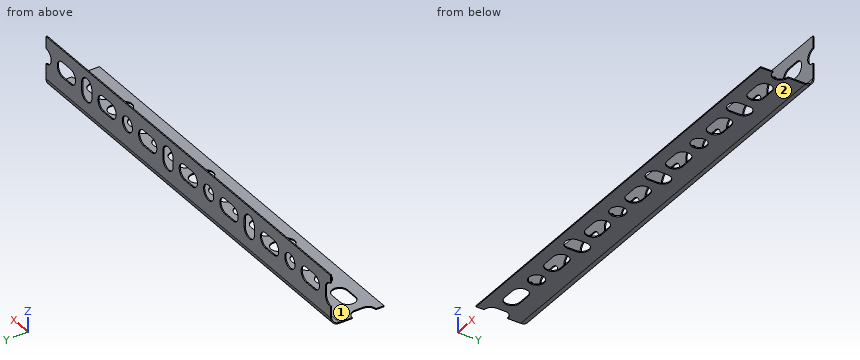
```python
from build123d import *

# Parameters (mm, degrees)
SKETCH1_W                    = 280
SKETCH1_H                    = 0.7366
BASE_FLANGE1_DEPTH           = 35
EDGE_FLANGE1_STRIP_W         = 12.9464
EDGE_FLANGE1_STRIP_H         = 0.7366
EDGE_FLANGE1_STRIP_CUT_DEPTH = 280
EDGE_FLANGE1_DEPTH           = 280
SKETCH11_R                   = 5
CUT_EXTRUDE1_DEPTH           = 149.199723952
LPATTERN1_COUNT              = 14
LPATTERN1_PITCH              = 80
SKETCH12_R                   = 5
CUT_EXTRUDE2_DEPTH           = 35
LPATTERN2_COUNT              = 15
LPATTERN2_PITCH              = 80


# Sheet-metal steps are written as plain solids
with BuildPart() as part:
    # Sketch1 → Base-Flange1 (new body)
    with BuildSketch(Plane(origin=(0, 0, 0), x_dir=(1, 0, 0), z_dir=(0, 1, 0))):
        with Locations((0, -0.3683)):
            Rectangle(SKETCH1_W, SKETCH1_H)
    extrude(amount=BASE_FLANGE1_DEPTH)

    # Edge-Flange1 strip (across the edge) → Edge-Flange1 strip cut (cut)
    with BuildSketch(Plane(origin=(140, 35, 0.7366), x_dir=(0, -1, 0), z_dir=(-1, 0, 0))):
        with Locations((-0.7366, -0.3683)):
            Rectangle(EDGE_FLANGE1_STRIP_W, EDGE_FLANGE1_STRIP_H)
    extrude(amount=EDGE_FLANGE1_STRIP_CUT_DEPTH, mode=Mode.SUBTRACT)

    # Edge-Flange1 section (across the edge) → Edge-Flange1 (add)
    with BuildSketch(Plane(origin=(140, 35, 0.7366), x_dir=(0, -1, 0), z_dir=(-1, 0, 0))):
        with BuildLine():
            Line((0, 5), (0, 33))
            Line((0, 33), (0.7366, 33))
            Line((0.7366, 33), (0.7366, 5))
            ThreePointArc((0.7366, 5), (2.201066094, 1.464466094), (5.7366, 0))
            Line((5.7366, 0), (5.7366, -0.7366))
            ThreePointArc((5.7366, -0.7366), (1.680211239, 0.943611239), (0, 5))
        make_face()
    extrude(amount=EDGE_FLANGE1_DEPTH)

    # Sketch11 → Cut-Extrude1 (cut, through all)
    with BuildSketch(Plane(origin=(0, 35, 0), x_dir=(1, 0, 0), z_dir=(0, 1, 0))):
        with Locations((140, -20.7366)):
            Circle(SKETCH11_R)
        with BuildLine():
            Line((124, -25.7366), (116, -25.7366))
            ThreePointArc((116, -25.7366), (111, -20.7366), (116, -15.7366))
            Line((116, -15.7366), (124, -15.7366))
            ThreePointArc((124, -15.7366), (129, -20.7366), (124, -25.7366))
        make_face()
        with BuildLine():
            Line((84, -25.7366), (76, -25.7366))
            ThreePointArc((76, -25.7366), (71, -20.7366), (76, -15.7366))
            Line((76, -15.7366), (84, -15.7366))
            ThreePointArc((84, -15.7366), (89, -20.7366), (84, -25.7366))
        make_face()
        with BuildLine():
            Line((95, -23.4866), (95, -17.9866))
            ThreePointArc((95, -17.9866), (100, -12.9866), (105, -17.9866))
            Line((105, -17.9866), (105, -23.4866))
            ThreePointArc((105, -23.4866), (100, -28.4866), (95, -23.4866))
        make_face()
    cut_extrude1 = extrude(amount=-CUT_EXTRUDE1_DEPTH, mode=Mode.SUBTRACT)

    # LPattern1: Cut-Extrude1 ×14
    with Locations(*[(-i * LPATTERN1_PITCH, 0, 0) for i in range(1, LPATTERN1_COUNT)]):
        add(cut_extrude1, mode=Mode.SUBTRACT)

    # Sketch12 → Cut-Extrude2 (cut)
    with BuildSketch(Plane.XY.offset(0.7366)):
        with Locations((140, 13)):
            Circle(SKETCH12_R)
        with BuildLine():
            Line((124, 8), (116, 8))
            ThreePointArc((116, 8), (111, 13), (116, 18))
            Line((116, 18), (124, 18))
            ThreePointArc((124, 18), (129, 13), (124, 8))
        make_face()
        with BuildLine():
            Line((95, 10.25), (95, 15.75))
            ThreePointArc((95, 15.75), (100, 20.75), (105, 15.75))
            Line((105, 15.75), (105, 10.25))
            ThreePointArc((105, 10.25), (100, 5.25), (95, 10.25))
        make_face()
        with BuildLine():
            Line((84, 8), (76, 8))
            ThreePointArc((76, 8), (71, 13), (76, 18))
            Line((76, 18), (84, 18))
            ThreePointArc((84, 18), (89, 13), (84, 8))
        make_face()
    cut_extrude2 = extrude(amount=-CUT_EXTRUDE2_DEPTH, mode=Mode.SUBTRACT)

    # LPattern2: Cut-Extrude2 ×15
    with Locations(*[(-i * LPATTERN2_PITCH, 0, 0) for i in range(1, LPATTERN2_COUNT)]):
        add(cut_extrude2, mode=Mode.SUBTRACT)


solid = part.part
```
The listing builds one solid part. Answer for the finished solid, in the listing's coordinates (mm). Face numbers are marked on the shaded views. A direction names the side the tool comes from. Round coordinates to 2 decimals unless told otherwise and drop trailing zeros. Write each loop counter-clockwise with the first axis right and the second up, starting at its lowest first coordinate (ties: lowest second). Pieces come first, ordered by that corner, then holes. Notation, with made-up numbers: (-1.75, 73.5) -> (55.25, 73.5) arc R22 ccw to (55.25, 102.5) -> close; hole circle Ø10 at (6.5, 72.25). An arc over 180 degrees is marked (long way). Use CSV: the item, a comma, the result in double quotes. Start each with the question number.
(1) Consider L1, parallel to Y at x = 64, z = 7.5; L2, parallel to Z at x = 0.5, y = 29; L3, parallel to Z at x = 1, y = 31.5. Determine where each line is inside the solid, lowest interval first. Write a range as from..to.
(2) Section A-A on x = -60 is taken. Give the vertices of the cut face in (y, z).
(3) Section C-C on x = -20 is taken. Give the vertices of the cut face in (y, z).
(4) Which of the six approach directions +Z, -Z, +X, -X, +Y, -Y give full straight-line access (tool end or side, diameter ignored) to the marked faces 1 and 2?
(5) Section D-D on y = 25 is taken. Give the vertices of the cut face in (x, z).
(6) Each of these flat-tipped pins is pushed along its axis until it touches: pin 1 (8 mm diameter, centred on x = 60, z = 20.74, fed in from -Y); pin 2 (0.6 mm diameter, centred on y = 35, z = 20.5, fed in from -X); pin 3 (5 mm diameter, centred on x = 78, y = 24.5, fed in from +Z); pin 4 (0.6 mm diameter, centred on x = -38, z = 0.5, fed in from +Y). Where does it stop, or does it pass through?
(7) Section B-B on y = 13 is taken. Count the separate pieces of the cut face and the enclosed holes in it, then the cut area to 3 significant figures.
A:
1,L1,"y = 34.26..35"
1,L2,"z = 0..0.74"
1,L3,"z = 0.45..1.26"
2,outline,"(0, 0) -> (5.25, 0) -> (5.25, 0.74) -> (0, 0.74) -> close; (20.75, 0) -> (29.26, 0) arc R5.74 ccw to (35, 5.74) -> (35, 12.99) -> (34.26, 12.99) -> (34.26, 5.74) arc R5 cw to (29.26, 0.74) -> (20.75, 0.74) -> close; (34.26, 28.49) -> (35, 28.49) -> (35, 33.74) -> (34.26, 33.74) -> close"
3,outline,"(0, 0) -> (8, 0) -> (8, 0.74) -> (0, 0.74) -> close; (18, 0) -> (29.26, 0) arc R5.74 ccw to (35, 5.74) -> (35, 15.74) -> (34.26, 15.74) -> (34.26, 5.74) arc R5 cw to (29.26, 0.74) -> (18, 0.74) -> close; (34.26, 25.74) -> (35, 25.74) -> (35, 33.74) -> (34.26, 33.74) -> close"
4,face 1,"+Z, +X, -X, -Y"
4,face 2,"-Z, +X, -X, +Y, -Y"
5,outline,"(-140, 0) -> (140, 0) -> (140, 0.74) -> (-140, 0.74) -> close"
6,pin 1,"passes through"
6,pin 2,"stops at x = -135"
6,pin 3,"stops at z = 0.74"
6,pin 4,"stops at y = 32.19"
7,separate pieces,"14"
7,enclosed holes,"0"
7,area,"61.9 mm²"
